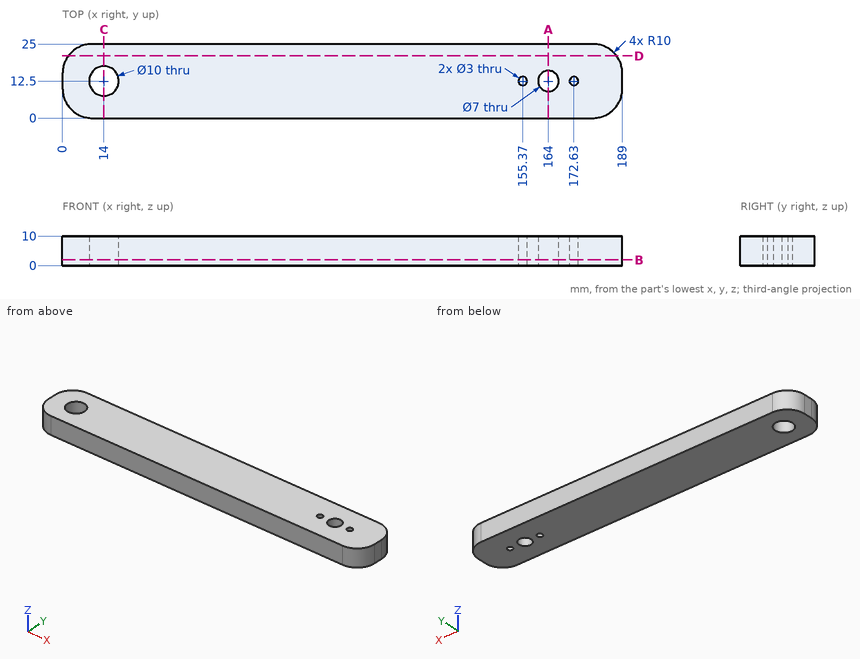
Design review of the part shown in the three views and the two pictorial views. Dimensions are in mm from the part's minimum x, y and z. Coordinates: 2 decimals unless noted, no trailing zeros. Order: outer loops, then holes, each group sorted by start corner. A loop starts at its lowest first (then second) coordinate and runs counter-clockwise, first axis right, second up. Notation, with made-up numbers: (-36.5, -30) - (-17.5, -30) arc R20 cw to (-17.5, -4) - close; hole circle Ø3 at (-1.75, 82.25). An arc over 180 degrees is marked (long way). Answer as CSV lines item,"result". Start each with the question number.
1) To check wall thickness, follow line 1 along Y through (x, z) = (164, 5.75); line 2 along Y through (x, z) = (172.63, 7.75); line 3 along X through (y, z) = (14.25, 6). State the ranges of each line that lie inside material, in increasing order. Write a range as [from, to].
2) Add section D-D (y = 21). State the section outline as (x, z) points.
3) Add section B-B (z = 2). State the section outline as (x, y) points.
4) Add section A-A (x = 164). State the section outline as (y, z) points.
5) Add section C-C (x = 14). State the section outline as (y, z) points.
6) Insertion check: P1, Ø5, axis at x = 172.63, y = 12.5, coming from the -Z side; P2, Ø1, axis at y = 20.5, z = 8.5, coming from the -X side; P3, Ø2, axis at y = 19, z = 3.5, coming from the +X side. Each pin has a flat end and moves straight along its axis. Give the tip position at first contact, or say it passes through.
Result:
1,line 1,"[0, 9], [16, 25]"
1,line 2,"[0, 11], [14, 25]"
1,line 3,"[0, 9.32], [18.68, 160.97], [167.03, 189]"
2,outline,"(2, 0) - (187, 0) - (187, 10) - (2, 10) - close"
3,outline,"(0, 10) arc R10 ccw to (10, 0) - (179, 0) arc R10 ccw to (189, 10) - (189, 15) arc R10 ccw to (179, 25) - (10, 25) arc R10 ccw to (0, 15) - close; hole circle Ø10 at (14, 12.5); hole circle Ø3 at (155.37, 12.5); hole circle Ø7 at (164, 12.5); hole circle Ø3 at (172.63, 12.5)"
4,outline,"(0, 0) - (9, 0) - (9, 10) - (0, 10) - close; (16, 0) - (25, 0) - (25, 10) - (16, 10) - close"
5,outline,"(0, 0) - (7.5, 0) - (7.5, 10) - (0, 10) - close; (17.5, 0) - (25, 0) - (25, 10) - (17.5, 10) - close"
6,P1,"z = 0"
6,P2,"x = 1.34"
6,P3,"x = 188.54"
